For this review, use the dimensioned drawing (mm, ordinates from the lowest corner) and the shaded views. Give positions to 0.01 mm unless a question says otherwise; leave off trailing zeros. Order: outer loops, then holes, each group sorted by start corner. A loop starts at its lowest first (then second) coordinate and runs counter-clockwise, first axis right, second up.
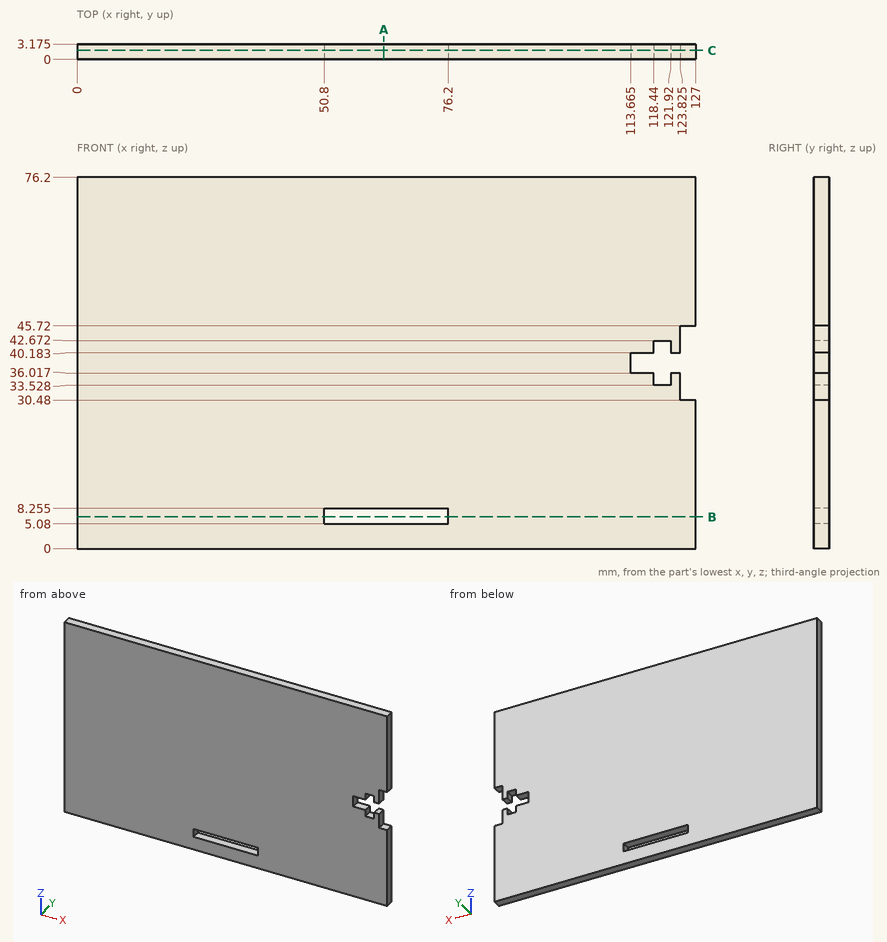
1. Take a section at B-B (z = 6.5). Write out the cut boundary in (x, y) (3 decimals).
2. Take a section at A-A (x = 63). Write out the cut boundary in (y, z) (3 decimals).
3. Take a section at C-C (y = 1.85). Write out the cut boundary in (x, z) (1 decimal).
4. Insertion check: pin 1 (1 mm diameter, centred on x = 56, z = 8.5, fed in from -Y); pin 2 (1.2 mm diameter, centred on y = 2, z = 41, fed in from +X) (3 decimals). Each pin has a flat end and moves straight along its axis. Give the tip position at first contact, or say it passes through.
5. To check wall thickness, follow line 1 (Z direction, x = 64, y = 2.85) (3 decimals); line 2 (X direction, y = 3, z = 33) (3 decimals). State the ranges of each line that lie inside material, in increasing order.
Answer:
1. outline: (0, 0) - (50.8, 0) - (50.8, 3.175) - (0, 3.175) - close; (76.2, 0) - (127, 0) - (127, 3.175) - (76.2, 3.175) - close
2. outline: (0, 0) - (3.175, 0) - (3.175, 5.08) - (0, 5.08) - close; (0, 8.255) - (3.175, 8.255) - (3.175, 76.2) - (0, 76.2) - close
3. outline: (0, 0) - (127, 0) - (127, 30.5) - (123.8, 30.5) - (123.8, 36) - (121.9, 36) - (121.9, 33.5) - (118.4, 33.5) - (118.4, 36) - (113.7, 36) - (113.7, 40.2) - (118.4, 40.2) - (118.4, 42.7) - (121.9, 42.7) - (121.9, 40.2) - (123.8, 40.2) - (123.8, 45.7) - (127, 45.7) - (127, 76.2) - (0, 76.2) - close; hole (50.8, 5.1) - (76.2, 5.1) - (76.2, 8.3) - (50.8, 8.3) - close
4. pin 1: stops at y = 0
4. pin 2: stops at x = 123.825
5. line 1: z = 0 to 5.08, 8.255 to 76.2
5. line 2: x = 0 to 123.825
